Geometry check sheet. Reference: the model listing, model coordinates, mm. A direction names the side the tool comes from. Give positions to 0.01 mm unless a question says otherwise; leave off trailing zeros. Loops run counter-clockwise (first coordinate to the right, second up) from the corner with the lowest first, then second, coordinate; pieces in that order, holes last. Notation, with made-up numbers: (47, 88) -> (80, 88) arc R12 cw to (80, 104) -> close; hole circle Ø9 at (16, -17.5). An arc over 180 degrees is marked (long way). One line per question, with ' | ' between items.
from build123d import *

# Parameters (mm, degrees)
SKETCH1_R                                        = 19.05
BOSS_EXTRUDE1_DEPTH                              = 15.875
FILLET2_R                                        = 3.175
FILLET3_R                                        = 4.7752
SKETCH6_R                                        = 36.5099981
CUT_EXTRUDE2_DEPTH                               = 2.54
CBORE_FOR_1_4_SOCKET_HEAD_CAP_SCREW1_D           = 6.5278
CBORE_FOR_1_4_SOCKET_HEAD_CAP_SCREW1_CBORE_D     = 11.1125
CBORE_FOR_1_4_SOCKET_HEAD_CAP_SCREW1_CBORE_DEPTH = 6.35
F_1_4_20_TAPPED_HOLE1_D                          = 5.1054
F_1_4_20_TAPPED_HOLE1_DEPTH                      = 19.05
F_1_4_20_TAPPED_HOLE1_CSINK_D                    = 6.3754
F_1_4_20_TAPPED_HOLE1_CSINK_ANGLE                = 90
F_1_4_20_TAPPED_HOLE1_TIP                        = 1.533816902


with BuildPart() as part:
    # Sketch1 → Boss-Extrude1 (new body)
    with BuildSketch(Plane(origin=(0, 0, 0), x_dir=(0, 0, -1), z_dir=(1, 0, 0))):
        with BuildLine():
            Line((-39.461181898, 44.45), (39.461181898, 44.45))
            ThreePointArc((39.461181898, 44.45), (41.955590949, 43.781625109), (43.781625109, 41.955590949))
            Line((43.781625109, 41.955590949), (61.588891971, 11.1125))
            ThreePointArc((61.588891971, 11.1125), (61.588891971, 1.5875), (53.34, -3.175))
            Line((53.34, -3.175), (44.45, -3.175))
            Line((44.45, -3.175), (44.45, -44.45))
            Line((44.45, -44.45), (-44.45, -44.45))
            Line((-44.45, -44.45), (-44.45, -3.175))
            Line((-44.45, -3.175), (-53.34, -3.175))
            ThreePointArc((-53.34, -3.175), (-61.588891971, 1.5875), (-61.588891971, 11.1125))
            Line((-61.588891971, 11.1125), (-43.781625109, 41.955590949))
            ThreePointArc((-43.781625109, 41.955590949), (-41.955590949, 43.781625109), (-39.461181898, 44.45))
        make_face()
        Circle(SKETCH1_R, mode=Mode.SUBTRACT)
    extrude(amount=BOSS_EXTRUDE1_DEPTH)

    # Fillet2
    fillet2_edges = [part.edges().sort_by_distance(p)[0] for p in [
        (7.9375, -3.175, 44.45),
        (7.9375, -3.175, -44.45),
    ]]
    fillet(fillet2_edges, radius=FILLET2_R)

    # Fillet3
    fillet3_edges = [part.edges().sort_by_distance(p)[0] for p in [
        (7.9375, -44.45, 44.45),
        (7.9375, -44.45, -44.45),
    ]]
    fillet(fillet3_edges, radius=FILLET3_R)

    # Sketch6 → Cut-Extrude2 (cut)
    with BuildSketch(Plane(origin=(15.875, 0, 0), x_dir=(0, 0, -1), z_dir=(1, 0, 0))):
        Circle(SKETCH6_R)
    extrude(amount=-CUT_EXTRUDE2_DEPTH, mode=Mode.SUBTRACT)

    # CBORE for 1/4 Socket Head Cap Screw1 (through all)
    with Locations(Plane(origin=(15.875, 0, 0), x_dir=(0, 0, -1), z_dir=(1, 0, 0))):
        with Locations((-53.34, 6.35), (53.34, 6.35), (0, 33.02)):
            CounterBoreHole(CBORE_FOR_1_4_SOCKET_HEAD_CAP_SCREW1_D / 2, CBORE_FOR_1_4_SOCKET_HEAD_CAP_SCREW1_CBORE_D / 2, CBORE_FOR_1_4_SOCKET_HEAD_CAP_SCREW1_CBORE_DEPTH)

    # 1/4-20 Tapped Hole1
    with Locations(Plane(origin=(15.875, 0, 0), x_dir=(0, 0, -1), z_dir=(1, 0, 0))):
        with Locations((34.8, -34.8), (-34.8, 34.8), (-34.8, -34.8), (34.8, 34.8)):
            CounterSinkHole(F_1_4_20_TAPPED_HOLE1_D / 2, F_1_4_20_TAPPED_HOLE1_CSINK_D / 2, depth=F_1_4_20_TAPPED_HOLE1_DEPTH, counter_sink_angle=F_1_4_20_TAPPED_HOLE1_CSINK_ANGLE)
            with Locations((0, 0, -(F_1_4_20_TAPPED_HOLE1_DEPTH + F_1_4_20_TAPPED_HOLE1_TIP / 2))):  # 118° drill point
                Cone(0, F_1_4_20_TAPPED_HOLE1_D / 2, F_1_4_20_TAPPED_HOLE1_TIP, mode=Mode.SUBTRACT)


solid = part.part
Item 1: Scan lines: probe 1 along Z at (x, y) = (5.5, -34.8); probe 2 along Z at (x, y) = (2.5, -35). Record each from-to range of solid material in increasing order.
Result:
probe 1: -44.45 to -37.35, -32.25 to 32.25, 37.35 to 44.45 | probe 2: -44.45 to -37.34, -32.26 to 32.26, 37.34 to 44.45
Item 2: Set-up check for faces 1 (the face through (12.04, 38.53, 0.72)), 2 (the face through (8, -3.175, 50)), 3 (the face through (8, -23, -44.45)): record each of +Z, -Z, +X, -X, +Y, -Y from which the full face is reachable in a straight line by a thin tool's end or side.
Result:
face 1: +X | face 2: +Z, +X, -X, -Y | face 3: -Z, +X, -X, -Y
Item 3: Sectioned sample at C-C (z = -16). Record the cut outline in (x, y) (3 decimals), plus the area to 3 significant figures.
Result:
outline: (0, -44.45) -> (15.875, -44.45) -> (15.875, -32.817) -> (13.335, -32.817) -> (13.335, -10.339) -> (0, -10.339) -> close; (0, 10.339) -> (13.335, 10.339) -> (13.335, 32.817) -> (15.875, 32.817) -> (15.875, 44.45) -> (0, 44.45) -> close | area: 969 mm2
Item 4: Release check for a two-part mould opening along Z. For faces 4 (the face through (8, -43, 43.1)), 5 (the face through (12.74, 4.22, -58.47)), 6 (the face through (7.513, -32.648, 36.172)), 7 (the face through (8, 44.45, 1)) record: pulls with the +Z half, pulls with the -Z half, needs draft (parallel to the pull), parting line crosses it, or undercut.
Result:
face 4: pulls with the +Z half | face 5: undercut | face 6: undercut | face 7: needs draft
Item 5: Sectioned sample at B-B (y = 15). Record the cut outline in (x, z) (3 decimals), plus the area to 3 significant figures.
Result:
outline: (0, -59.344) -> (15.875, -59.344) -> (15.875, -33.286) -> (13.335, -33.286) -> (13.335, -11.743) -> (0, -11.743) -> close; (0, 11.743) -> (13.335, 11.743) -> (13.335, 33.286) -> (15.875, 33.286) -> (15.875, 59.344) -> (0, 59.344) -> close | area: 1,400 mm2
Item 6: Sectioned sample at A-A (x = 6). Give the number of separate pieces and of enclosed holes in the cut face, plus the area to 3 significant figures.
Result:
separate pieces: 1 | enclosed holes: 8 | area: 7,560 mm2
Item 7: Depth check by flat-ended pin: pin 1 Ø4 at (y, z) = (-30, -4) entering from +X (3 decimals); pin 2 Ø3 at (y, z) = (34.8, 34.8) entering from -X; pin 3 Ø7.5 at (y, z) = (33.02, 0) entering from +X (3 decimals); pin 4 Ø8 at (x, y) = (7.5, -27) entering from -Z. Enter the tip coordinate at first touch or a pass-through.
Result:
pin 1: x = 13.335 | pin 2: through | pin 3: x = 9.525 | pin 4: z = -44.45
